Can you work these out from the model? Positions are in its coordinate system, mm. Face numbers are marked on the shaded views. Round coordinates to 2 decimals unless told otherwise and drop trailing zeros. Order: outer loops, then holes, each group sorted by start corner. A loop starts at its lowest first (then second) coordinate and runs counter-clockwise, first axis right, second up. Notation, with made-up numbers: M 7,22.25 L 64,22.25 A26 cw 64,56.25 Z; hole C 35,0.5 d11. An arc over 180 degrees is marked long. Answer as a JSON object with one key per item and string values. Group by question number.
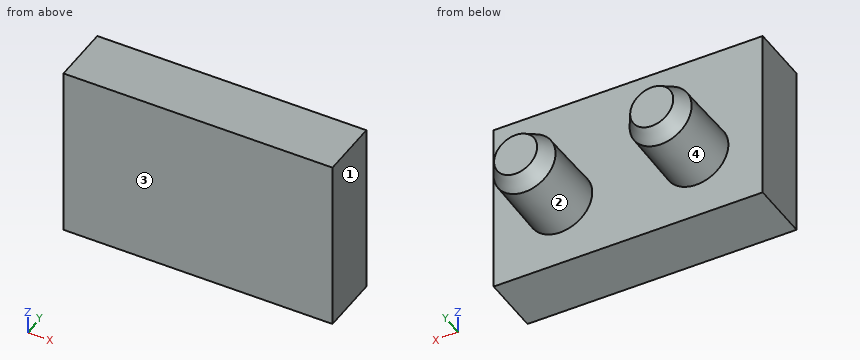
from build123d import *
from OCP.BRepFilletAPI import BRepFilletAPI_MakeChamfer

# Parameters (mm, degrees)
SKETCH1_W                     = 8.5
SKETCH1_H                     = 5.5
BOSS_EXTRUDE1_DEPTH           = 1.9
BOSS_EXTRUDE2_REACH           = 8.307
BOSS_EXTRUDE2_START           = 0.9
SKETCH2_R                     = 1
BOSS_EXTRUDE2_DRAFT           = 1
BOSS_EXTRUDE3_START           = 0.9
SKETCH2_2_R                   = 1
BOSS_EXTRUDE3_DEPTH           = 1.6
BOSS_EXTRUDE3_DRAFT           = 1
BOSS_EXTRUDE3_PROFILE_2_DEPTH = 1.6
BOSS_EXTRUDE3_PROFILE_2_DRAFT = 1
CHAMFER1_SIZE                 = 0.5
CHAMFER1_SIZE2                = 0.291658349


with BuildPart() as part:
    # Sketch1 → Boss-Extrude1 (new body)
    with BuildSketch(Plane(origin=(0, 0, 0), x_dir=(1, 0, 0), z_dir=(0, 1, 0))):
        Rectangle(SKETCH1_W, SKETCH1_H)
    extrude(amount=BOSS_EXTRUDE1_DEPTH)




with BuildPart() as boss_extrude2_long_prism_1:
    # Sketch2 → Boss-Extrude2 (the long prism of profile 1, to be tilted and cut off)
    with BuildSketch(Plane(origin=(0, 1.9, 0), x_dir=(1, 0, 0), z_dir=(0, 1, 0)).offset(BOSS_EXTRUDE2_START)):
        with Locations((-2.15, 0.65)):
            Circle(SKETCH2_R)
    extrude(amount=-BOSS_EXTRUDE2_REACH)
    boss_extrude2_tool1_sides = [boss_extrude2_long_prism_1.faces().sort_by_distance(p)[0] for p in [
        (-3.15, -1.3535, -0.65),
    ]]
    draft(boss_extrude2_tool1_sides, Plane(origin=(0, 1.9, 0), x_dir=(1, 0, 0), z_dir=(0, 1, 0)).offset(BOSS_EXTRUDE2_START), BOSS_EXTRUDE2_DRAFT)  # the draft: side faces tilted about the start plane


with BuildPart() as part_1:
    add(part.part)
    boss_extrude2_tool1 = boss_extrude2_long_prism_1.part - part.part



with BuildPart() as boss_extrude2_long_prism_2:
    # Sketch2 → Boss-Extrude2 (the long prism of profile 2, to be tilted and cut off)
    with BuildSketch(Plane(origin=(0, 1.9, 0), x_dir=(1, 0, 0), z_dir=(0, 1, 0)).offset(BOSS_EXTRUDE2_START)):
        with Locations((2.15, 0.65)):
            Circle(SKETCH2_R)
    extrude(amount=-BOSS_EXTRUDE2_REACH)
    boss_extrude2_tool2_sides = [boss_extrude2_long_prism_2.faces().sort_by_distance(p)[0] for p in [
        (1.15, -1.3535, -0.65),
    ]]
    draft(boss_extrude2_tool2_sides, Plane(origin=(0, 1.9, 0), x_dir=(1, 0, 0), z_dir=(0, 1, 0)).offset(BOSS_EXTRUDE2_START), BOSS_EXTRUDE2_DRAFT)  # the draft: side faces tilted about the start plane


with BuildPart() as part_2:
    add(part_1.part)
    boss_extrude2_tool2 = boss_extrude2_long_prism_2.part - part.part
    add(boss_extrude2_tool1.solids().sort_by_distance((-2.15, 2.8, -0.65))[0])
    add(boss_extrude2_tool2.solids().sort_by_distance((2.15, 2.8, -0.65))[0])


with BuildPart() as boss_extrude3_tool:
    # Sketch2<2> → Boss-Extrude3 (with draft: the straight prism first)
    with BuildSketch(Plane(origin=(0, 1.9, 0), x_dir=(1, 0, 0), z_dir=(0, 1, 0)).offset(BOSS_EXTRUDE3_START)):
        with Locations((-2.15, 0.65)):
            Circle(SKETCH2_2_R)
    extrude(amount=BOSS_EXTRUDE3_DEPTH)
    # Boss-Extrude3: the draft: its side faces are tilted about the plane it starts from
    boss_extrude3_sides = [boss_extrude3_tool.faces().sort_by_distance(p)[0] for p in [
        (-3.15, 3.6, -0.65),
    ]]
    draft(boss_extrude3_sides, Plane(origin=(0, 1.9, 0), x_dir=(1, 0, 0), z_dir=(0, 1, 0)).offset(BOSS_EXTRUDE3_START), BOSS_EXTRUDE3_DRAFT)


with BuildPart() as part_3:
    add(part_2.part)

    # Boss-Extrude3: add boss_extrude3_tool
    add(boss_extrude3_tool.part)


with BuildPart() as boss_extrude3_profile_2_tool:
    # Sketch2<2> → Boss-Extrude3 profile 2 (with draft: the straight prism first)
    with BuildSketch(Plane(origin=(0, 1.9, 0), x_dir=(1, 0, 0), z_dir=(0, 1, 0)).offset(BOSS_EXTRUDE3_START)):
        with Locations((2.15, 0.65)):
            Circle(SKETCH2_2_R)
    extrude(amount=BOSS_EXTRUDE3_PROFILE_2_DEPTH)
    # Boss-Extrude3 profile 2: the draft: its side faces are tilted about the plane it starts from
    boss_extrude3_profile_2_sides = [boss_extrude3_profile_2_tool.faces().sort_by_distance(p)[0] for p in [
        (1.15, 3.6, -0.65),
    ]]
    draft(boss_extrude3_profile_2_sides, Plane(origin=(0, 1.9, 0), x_dir=(1, 0, 0), z_dir=(0, 1, 0)).offset(BOSS_EXTRUDE3_START), BOSS_EXTRUDE3_PROFILE_2_DRAFT)


with BuildPart() as part_4:
    add(part_3.part)

    # Boss-Extrude3 profile 2: add boss_extrude3_profile_2_tool
    add(boss_extrude3_profile_2_tool.part)

    # Chamfer1: one chamfer whose edges measure the first distance from different faces: ONE call of the kernel's chamfer builder (chamfer() names one face for all edges)
    chamfer1_edges_1 = [part_4.edges().sort_by_distance(p)[0] for p in [
        (-3.122071896, 4.4, -0.65),
    ]]
    chamfer1_side_1 = [part_4.faces().sort_by_distance(p)[0] for p in [
        (-3.143890727, 3.15, -0.65),
    ]]
    chamfer1_edges_2 = [part_4.edges().sort_by_distance(p)[0] for p in [
        (1.177928104, 4.4, -0.65),
    ]]
    chamfer1_side_2 = [part_4.faces().sort_by_distance(p)[0] for p in [
        (1.156109273, 3.15, -0.65),
    ]]
    chamfer1 = BRepFilletAPI_MakeChamfer(part_4.part.solid().wrapped)
    for e in chamfer1_edges_1:
        chamfer1.Add(CHAMFER1_SIZE, CHAMFER1_SIZE2, e.wrapped, chamfer1_side_1[0].wrapped)  # the first distance lies on this face
    for e in chamfer1_edges_2:
        chamfer1.Add(CHAMFER1_SIZE, CHAMFER1_SIZE2, e.wrapped, chamfer1_side_2[0].wrapped)  # the first distance lies on this face
    add(Compound.cast(chamfer1.Shape()), mode=Mode.REPLACE)


solid = part_4.part
Item 1: Suppose I cut it at A-A, the plane z = 1.7. Write out the boundary of the cut face in (x, y).
Item 2: I need wall thicknesses on line 1 (Y direction, x = -3.25, z = 0.95); line 2 (Z direction, x = -2.25, y = 3.6); line 3 (X direction, y = 2.7, z = -0.3). Which ranges of each line are inside material? Lowest first, please.
Item 3: If we mould it in two halves opening along X, with no side actions, what happens to the marked faces 1, 2, 3 and 4? For each: +X half, -X half, draft (parallel to the pull), parting line (faces both ways), or undercut.
Item 4: I'm going to push a flat-ended pin straight in: pin 1 Ø2 at (x, y) = (0.5, 4) entering from -Z. Where does the tip first touch, or does it pass through?
Item 5: Suppose I cut it at B-B, the plane x = 0.75. Write out the boundary of the cut face in (y, z).
Computed:
{
 "1": {"outline": "M -4.25,0 L 4.25,0 L 4.25,1.9 L -4.25,1.9 Z"},
 "2": {"line 1": "y = 0 to 1.9", "line 2": "z = -1.63 to 0.33", "line 3": "x = -3.09 to -1.21, 1.21 to 3.09"},
 "3": {"face 1": "+X half", "face 2": "undercut", "face 3": "draft", "face 4": "undercut"},
 "4": {"pin 1": "stops at z = -1.38"},
 "5": {"outline": "M 0,-2.75 L 1.9,-2.75 L 1.9,2.75 L 0,2.75 Z"}
}
